Design review of the part built by this model. Coordinates are the model's own, in mm. Coordinates: 2 decimals unless noted, no trailing zeros. Write each loop counter-clockwise with the first axis right and the second up, starting at its lowest first coordinate (ties: lowest second). Pieces come first, ordered by that corner, then holes. Notation, with made-up numbers: (13.5, 57) - (24.5, 57) arc R17 cw to (24.5, 89) - close; hole circle Ø4 at (67.5, 74). An arc over 180 degrees is marked (long way). Answer as CSV lines item,"result". Start each with the question number.
Q1. For line 1 along Z through (x, y) = (0.5, -19); line 2 along X through (y, z) = (-22.5, 4); line 3 along X through (y, z) = (-33, -6), list the stretches that pass through material, from the lowest coordinate up. Write a range as [from, to].
Q2. We need section B-B (z = 0). Write out the cut boundary in (x, y) (3 decimals), plus the area to 3 significant figures.
Q3. We need section C-C (y = -48.5). Write out the cut boundary in (x, z), plus the area to 3 significant figures.
Q4. We need section A-A (x = 0). Write out the cut boundary in (y, z) (3 decimals), plus the area to 3 significant figures.
from build123d import *

# Parameters (mm, degrees)
F0_R     = 12.7
F1_DEPTH = 56.515


with BuildPart() as f1:
    # F0 (on Front) → F1 (new body)
    with BuildSketch(Plane.XZ):
        with BuildLine():
            ThreePointArc((-3.8e-08, -31.75), (22.4506402893, -22.4506403161), (31.75, 0))
            ThreePointArc((31.75, 0), (22.4506402996, 22.4506403057), (-8.6e-09, 31.75))
            ThreePointArc((-8.6e-09, 31.75), (-22.4506403095, 22.4506402959), (-31.75, -1.06e-08))
            ThreePointArc((-31.75, -1.06e-08), (-22.4506403123, -22.450640293), (-3.8e-08, -31.75))
        make_face()
        Circle(F0_R, mode=Mode.SUBTRACT)
        with BuildLine():
            Line((31.75, -31.75), (31.75, 0))
            ThreePointArc((31.75, 0), (22.4506402893, -22.4506403161), (-3.8e-08, -31.75))
            Line((-3.8e-08, -31.75), (31.75, -31.75))
        make_face()
        with BuildLine():
            ThreePointArc((-8.6e-09, 31.75), (22.4506402996, 22.4506403057), (31.75, 0))
            Line((31.75, 0), (31.75, 31.75))
            Line((31.75, 31.75), (-8.6e-09, 31.75))
        make_face()
        with BuildLine():
            ThreePointArc((-31.75, -1.06e-08), (-22.4506403095, 22.4506402959), (-8.6e-09, 31.75))
            Line((-8.6e-09, 31.75), (-31.75, 31.75))
            Line((-31.75, 31.75), (-31.75, -1.06e-08))
        make_face()
        with BuildLine():
            Line((-31.75, -31.75), (-3.8e-08, -31.75))
            ThreePointArc((-3.8e-08, -31.75), (-22.4506403123, -22.450640293), (-31.75, -1.06e-08))
            Line((-31.75, -1.06e-08), (-31.75, -31.75))
        make_face()
    extrude(amount=F1_DEPTH)


solid = f1.part
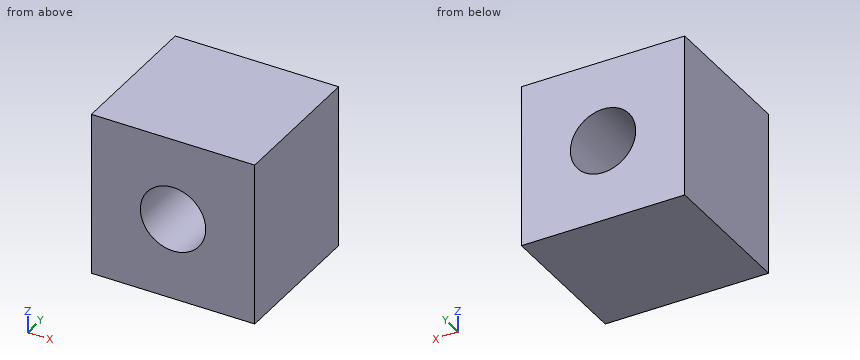
Results list:
1,line 1,"z = [-31.75, -12.69], [12.69, 31.75]"
1,line 2,"x = [-31.75, -12.05], [12.05, 31.75]"
1,line 3,"x = [-31.75, -11.19], [11.19, 31.75]"
2,outline,"(-31.75, -56.515) - (-12.7, -56.515) - (-12.7, 0) - (-31.75, 0) - close; (12.7, -56.515) - (31.75, -56.515) - (31.75, 0) - (12.7, 0) - close"
2,area,"2,150 mm2"
3,outline,"(-31.75, -31.75) - (31.75, -31.75) - (31.75, 31.75) - (-31.75, 31.75) - close; hole circle Ø25.4 at (0, 0)"
3,area,"3,530 mm2"
4,outline,"(-56.515, -31.75) - (0, -31.75) - (0, -12.7) - (-56.515, -12.7) - close; (-56.515, 12.7) - (0, 12.7) - (0, 31.75) - (-56.515, 31.75) - close"
4,area,"2,150 mm2"
